Verification items for this drawing (mm, ordinates from the low corner). A direction names the side the tool comes from. Round coordinates to 2 decimals unless told otherwise and drop trailing zeros. Order: outer loops, then holes, each group sorted by start corner. A loop starts at its lowest first (then second) coordinate and runs counter-clockwise, first axis right, second up. Notation, with made-up numbers: (44, -1.75) -> (68, -1.75) arc R11 ccw to (68, 10.25) -> close; hole circle Ø8 at (17.5, 39). An arc over 180 degrees is marked (long way). Put each result on its own line as item: value.
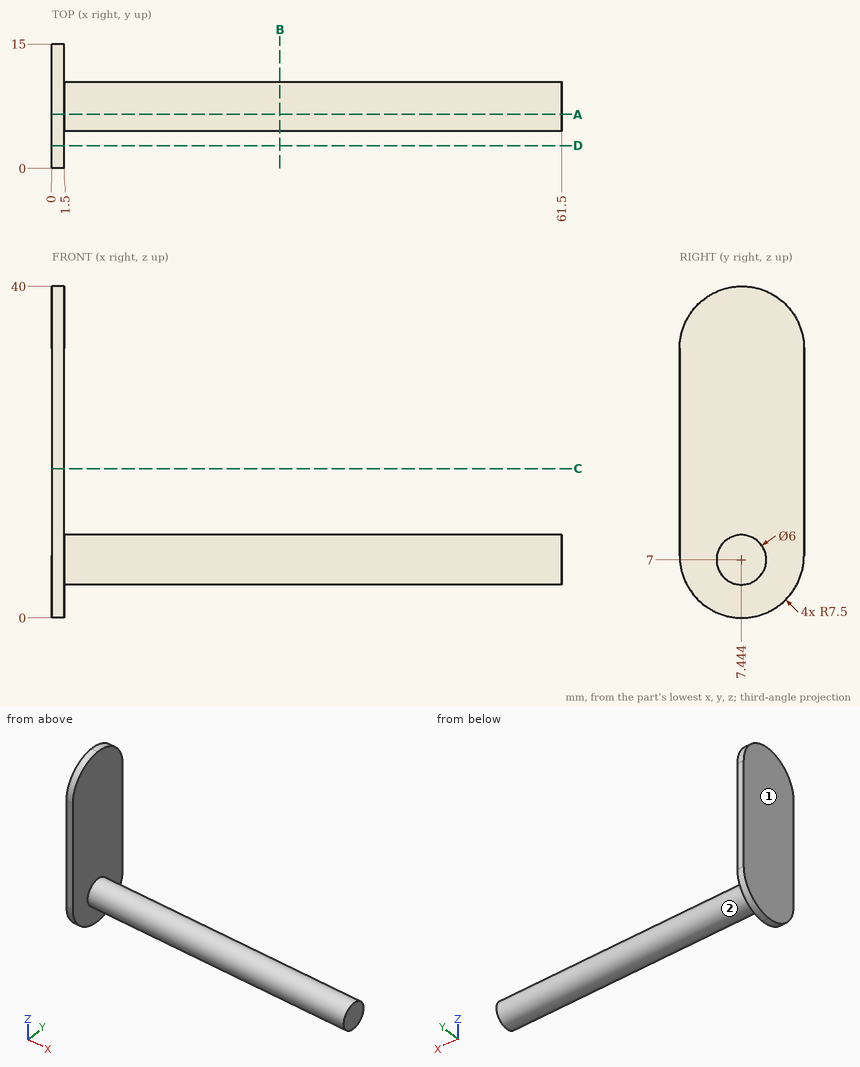
Item 1: Gauge pin test, flat ends, axial feed: pin 1 Ø6 at (x, y) = (32.5, 10.5) entering from +Z; pin 2 Ø1 at (y, z) = (9, 15.5) entering from +X. Record the tip position at first contact, or that the pin passes through.
Check sheet entries:
pin 1: stops at z = 10
pin 2: stops at x = 1.5
Item 2: Section check B-B on x = 27.5. Record the boundary of the cut face in (y, z), then the cut area to 3 significant figures.
Check sheet entries:
outline: circle Ø6 at (7.44, 7)
area: 28.3 mm^2
Item 3: Section check A-A on y = 6.5. Record the boundary of the cut face in (x, z).
Check sheet entries:
outline: (0, 0.07) -> (1.5, 0.07) -> (1.5, 4.15) -> (61.5, 4.15) -> (61.5, 9.85) -> (1.5, 9.85) -> (1.5, 39.93) -> (0, 39.93) -> close
Item 4: Material ranges on L1, parallel to X at y = 11, z = 36.5; L2, parallel to Z at x = 50.5, y = 9.5 (1 decimal); L3, parallel to Z at x = 37.5, y = 9 (1 decimal), recorded low to high. Write a range as [from, to].
Check sheet entries:
L1: x = [0, 1.5]
L2: z = [4.8, 9.2]
L3: z = [4.4, 9.6]
Item 5: Section check C-C on z = 18. Record the boundary of the cut face in (x, y), then the cut area to 3 significant figures.
Check sheet entries:
outline: (0, 0) -> (1.5, 0) -> (1.5, 15) -> (0, 15) -> close
area: 22.5 mm^2
Item 6: Section check D-D on y = 2.75. Record the boundary of the cut face in (x, z).
Check sheet entries:
outline: (0, 1.7) -> (1.5, 1.7) -> (1.5, 38.3) -> (0, 38.3) -> close
Item 7: Tool access check on the marked faces 1 and 2. Record the directions out of +Z, -Z, +X, -X, +Y, -Y that give a thin tool (end or side, any length) a straight path to the whole face; none if there is none.
Check sheet entries:
face 1: +Z, -Z, -X, +Y, -Y
face 2: +X
